Can you work these out from the model? Positions are in its coordinate system, mm. Face numbers are marked on the shaded views. A direction names the side the tool comes from. Give positions to 0.01 mm unless a question says otherwise; leave off trailing zeros. Write each loop counter-clockwise with the first axis right and the second up, starting at its lowest first coordinate (ties: lowest second). Pieces come first, ordered by that corner, then holes. Notation, with made-up numbers: (13, 44.25) - (47, 44.25) arc R13 cw to (47, 63.25) - close; hole circle Ø1 at (48.25, -18.5). An arc over 180 degrees is marked (long way). Return JSON: item names as keys, results as strings. Group by question number.
from build123d import *

# Parameters (mm, degrees)
RESSALTO_EXTRUS_O2_DEPTH      = 30
RESSALTO_EXTRUS_O3_START      = 3
RESSALTO_EXTRUS_O3_DEPTH      = 3
RESSALTO_EXTRUS_O4_DEPTH      = 3
RESSALTO_EXTRUS_O4_DEPTH_BACK = 10
CORTE_EXTRUS_O1_DEPTH         = 10
CORTE_EXTRUS_O2_REACH         = 83.702
FILETE1_START                 = -19.773073923
FILETE1_DEPTH                 = 36.75
FILETE1_START_2               = -13.40159992
FILETE1_2_DEPTH               = 59
ESBO_O10_R                    = 1.5
CORTE_EXTRUS_O3_DEPTH         = 10
CORTE_EXTRUS_O4_DEPTH         = 10
FILETE2_R                     = 2


with BuildPart() as part:
    # Esboço2 → Ressalto-extrusão2 (new body)
    with BuildSketch(Plane(origin=(0, 0, 0), x_dir=(0, 0, -1), z_dir=(1, 0, 0))):
        with BuildLine():
            Line((2.90159992, -0.062465938), (-35.09840008, -0.062465938))
            Line((-35.09840008, -0.062465938), (-39.886084903, -0.062465938))
            ThreePointArc((-39.886084903, -0.062465938), (-45.202180234, 1.467638524), (-48.891439328, 5.589707975))
            ThreePointArc((-48.891439328, 5.589707975), (-52.096536948, 9.772081499), (-56.69840008, 12.338743681))
            ThreePointArc((-56.69840008, 12.338743681), (-59.373224015, 11.895603401), (-60.59840008, 9.476926077))
            Line((-60.59840008, 9.476926077), (-60.59840008, 20.976926077))
            ThreePointArc((-60.59840008, 20.976926077), (-59.719720424, 23.09824642), (-57.59840008, 23.976926077))
            Line((-57.59840008, 23.976926077), (25.40159992, 23.976926077))
            ThreePointArc((25.40159992, 23.976926077), (27.522920263, 23.09824642), (28.40159992, 20.976926077))
            Line((28.40159992, 20.976926077), (28.40159992, 9.476926077))
            ThreePointArc((28.40159992, 9.476926077), (27.176423855, 11.895603401), (24.50159992, 12.338743681))
            ThreePointArc((24.50159992, 12.338743681), (19.899736788, 9.772081499), (16.694639168, 5.589707975))
            ThreePointArc((16.694639168, 5.589707975), (13.005380073, 1.467638524), (7.689284743, -0.062465938))
            Line((7.689284743, -0.062465938), (2.90159992, -0.062465938))
        make_face()
    extrude(amount=RESSALTO_EXTRUS_O2_DEPTH)

    # Esboço3 → Ressalto-extrusão3 (add)
    with BuildSketch(Plane.ZY.offset(RESSALTO_EXTRUS_O3_START)):
        with BuildLine():
            Line((60.59840008, 15.226926077), (60.59840008, 20.976926077))
            ThreePointArc((60.59840008, 20.976926077), (59.719720424, 23.09824642), (57.59840008, 23.976926077))
            Line((57.59840008, 23.976926077), (16.09840008, 23.976926077))
            Line((16.09840008, 23.976926077), (-25.40159992, 23.976926077))
            ThreePointArc((-25.40159992, 23.976926077), (-27.522920263, 23.09824642), (-28.40159992, 20.976926077))
            Line((-28.40159992, 20.976926077), (-28.40159992, 15.226926077))
            Line((-28.40159992, 15.226926077), (-28.40159992, -16.773073923))
            ThreePointArc((-28.40159992, -16.773073923), (-27.522920263, -18.894394267), (-25.40159992, -19.773073923))
            Line((-25.40159992, -19.773073923), (57.59840008, -19.773073923))
            ThreePointArc((57.59840008, -19.773073923), (59.719720424, -18.894394267), (60.59840008, -16.773073923))
            Line((60.59840008, -16.773073923), (60.59840008, 15.226926077))
        make_face()
    extrude(amount=-RESSALTO_EXTRUS_O3_DEPTH)

    # Esboço4 → Ressalto-extrusão4 (add, two sides: drawn at the far end of the back side and taken through both)
    with BuildSketch(Plane(origin=(30, 0, 0), x_dir=(0, 0, -1), z_dir=(1, 0, 0)).offset(-RESSALTO_EXTRUS_O4_DEPTH_BACK)):
        with BuildLine():
            Line((-16.09840008, 23.976926077), (25.40159992, 23.976926077))
            ThreePointArc((25.40159992, 23.976926077), (27.522920263, 23.09824642), (28.40159992, 20.976926077))
            Line((28.40159992, 20.976926077), (28.40159992, 15.226926077))
            Line((28.40159992, 15.226926077), (28.40159992, -16.773073923))
            ThreePointArc((28.40159992, -16.773073923), (27.522920263, -18.894394267), (25.40159992, -19.773073923))
            Line((25.40159992, -19.773073923), (-57.59840008, -19.773073923))
            ThreePointArc((-57.59840008, -19.773073923), (-59.719720424, -18.894394267), (-60.59840008, -16.773073923))
            Line((-60.59840008, -16.773073923), (-60.59840008, 15.226926077))
            Line((-60.59840008, 15.226926077), (-60.59840008, 20.976926077))
            ThreePointArc((-60.59840008, 20.976926077), (-59.719720424, 23.09824642), (-57.59840008, 23.976926077))
            Line((-57.59840008, 23.976926077), (-16.09840008, 23.976926077))
        make_face()
    extrude(amount=RESSALTO_EXTRUS_O4_DEPTH + RESSALTO_EXTRUS_O4_DEPTH_BACK)

    # Esboço8 → Corte-extrusão1 (cut)
    with BuildSketch(Plane(origin=(33, 0, 0), x_dir=(0, 0, -1), z_dir=(1, 0, 0))):
        with BuildLine():
            Line((-43.59840008, -2.773073923), (11.40159992, -2.773073923))
            ThreePointArc((11.40159992, -2.773073923), (12.815813482, -3.358860361), (13.40159992, -4.773073923))
            Line((13.40159992, -4.773073923), (13.40159992, -10.773073923))
            ThreePointArc((13.40159992, -10.773073923), (12.815813482, -12.187287486), (11.40159992, -12.773073923))
            Line((11.40159992, -12.773073923), (-43.59840008, -12.773073923))
            ThreePointArc((-43.59840008, -12.773073923), (-45.012613643, -12.187287486), (-45.59840008, -10.773073923))
            Line((-45.59840008, -10.773073923), (-45.59840008, -4.773073923))
            ThreePointArc((-45.59840008, -4.773073923), (-45.012613643, -3.358860361), (-43.59840008, -2.773073923))
        make_face()
        with BuildLine():
            Line((-43.59840008, 6.976926077), (11.40159992, 6.976926077))
            ThreePointArc((11.40159992, 6.976926077), (12.815813482, 7.562712514), (13.40159992, 8.976926077))
            Line((13.40159992, 8.976926077), (13.40159992, 14.976926077))
            ThreePointArc((13.40159992, 14.976926077), (12.815813482, 16.391139639), (11.40159992, 16.976926077))
            Line((11.40159992, 16.976926077), (-43.59840008, 16.976926077))
            ThreePointArc((-43.59840008, 16.976926077), (-45.012613643, 16.391139639), (-45.59840008, 14.976926077))
            Line((-45.59840008, 14.976926077), (-45.59840008, 8.976926077))
            ThreePointArc((-45.59840008, 8.976926077), (-45.012613643, 7.562712514), (-43.59840008, 6.976926077))
        make_face()
    extrude(amount=-CORTE_EXTRUS_O1_DEPTH, mode=Mode.SUBTRACT)

    # Corte-extrusão2: up to this face of the body (flat: up to its plane)
    corte_extrus_o2_end = Plane(part.part.faces().sort_by_distance((28, 16.976926077, 16.09840008))[0])
    # Esboço9 → Corte-extrusão2 (cut, up to the picked face)
    with BuildSketch(Plane(origin=(0, -19.773073923, 0), x_dir=(-1, 0, 0), z_dir=(0, -1, 0)), mode=Mode.PRIVATE) as corte_extrus_o2_sk1:
        with BuildLine():
            Line((-25, 13.40159992), (-28, 13.40159992))
            ThreePointArc((-28, 13.40159992), (-29.414213562, 12.815813482), (-30, 11.40159992))
            Line((-30, 11.40159992), (-30, -43.59840008))
            ThreePointArc((-30, -43.59840008), (-29.414213562, -45.012613643), (-28, -45.59840008))
            Line((-28, -45.59840008), (-25, -45.59840008))
            ThreePointArc((-25, -45.59840008), (-23.585786438, -45.012613643), (-23, -43.59840008))
            Line((-23, -43.59840008), (-23, 11.40159992))
            ThreePointArc((-23, 11.40159992), (-23.585786438, 12.815813482), (-25, 13.40159992))
        make_face()
    corte_extrus_o2_tool1 = split(extrude(corte_extrus_o2_sk1.sketch, amount=-CORTE_EXTRUS_O2_REACH, mode=Mode.PRIVATE), bisect_by=corte_extrus_o2_end, keep=Keep.BOTH, mode=Mode.PRIVATE)
    add(corte_extrus_o2_tool1.solids().sort_by(Axis((26.5, -19.773074, 16.0984), (0, 1, 0)))[0], mode=Mode.SUBTRACT)

    # Filete1: read off the stored shape, not the designer's step
    # Filete1 outline → Filete1 (add)
    with BuildSketch(Plane(origin=(0, 0, 0), x_dir=(1, 0, 0), z_dir=(0, 1, 0)).offset(FILETE1_START)):
        with BuildLine():
            ThreePointArc((25, -45.59840008), (23.585786437, -45.012613642), (23, -43.59840008))
            Line((23, -43.59840008), (23, -45.59840008))
            Line((23, -45.59840008), (25, -45.59840008))
        make_face()
        with BuildLine():
            ThreePointArc((23, 11.40159992), (23.585786438, 12.815813482), (25, 13.40159992))
            Line((25, 13.40159992), (23, 13.40159992))
            Line((23, 13.40159992), (23, 11.40159992))
        make_face()
    extrude(amount=FILETE1_DEPTH)

    # Filete1 2 outline → Filete1 2 (add)
    with BuildSketch(Plane.XY.offset(FILETE1_START_2)):
        with BuildLine():
            ThreePointArc((23, 14.976926077), (23.585786438, 16.391139639), (25, 16.976926077))
            Line((25, 16.976926077), (23, 16.976926077))
            Line((23, 16.976926077), (23, 14.976926077))
        make_face()
    extrude(amount=FILETE1_2_DEPTH)

    # Esboço10 → Corte-extrusão3 (cut)
    with BuildSketch(Plane(origin=(0, 0, 0), x_dir=(0, 0, -1), z_dir=(1, 0, 0))):
        with Locations((-55.59840008, 6.338743681)):
            Circle(ESBO_O10_R)
        with Locations((23.40159992, 6.338743681)):
            Circle(ESBO_O10_R)
        with Locations((-16.09840008, -8.562465938)):
            Circle(ESBO_O10_R)
    extrude(amount=-CORTE_EXTRUS_O3_DEPTH, mode=Mode.SUBTRACT)

    # Esboço12 → Corte-extrusão4 (cut)
    with BuildSketch(Plane(origin=(0, 0, 0), x_dir=(0, 0, -1), z_dir=(1, 0, 0))):
        with BuildLine():
            Line((-31.59840008, -2.862465938), (-25.59840008, -2.862465938))
            ThreePointArc((-25.59840008, -2.862465938), (-24.184186518, -3.448252375), (-23.59840008, -4.862465938))
            Line((-23.59840008, -4.862465938), (-23.59840008, -14.773073923))
            ThreePointArc((-23.59840008, -14.773073923), (-24.184186518, -16.187287486), (-25.59840008, -16.773073923))
            Line((-25.59840008, -16.773073923), (-31.59840008, -16.773073923))
            ThreePointArc((-31.59840008, -16.773073923), (-33.012613643, -16.187287486), (-33.59840008, -14.773073923))
            Line((-33.59840008, -14.773073923), (-33.59840008, -4.862465938))
            ThreePointArc((-33.59840008, -4.862465938), (-33.012613643, -3.448252375), (-31.59840008, -2.862465938))
        make_face()
        with BuildLine():
            Line((-6.59840008, -2.862465938), (-0.59840008, -2.862465938))
            ThreePointArc((-0.59840008, -2.862465938), (0.815813482, -3.448252375), (1.40159992, -4.862465938))
            Line((1.40159992, -4.862465938), (1.40159992, -14.773073923))
            ThreePointArc((1.40159992, -14.773073923), (0.815813482, -16.187287486), (-0.59840008, -16.773073923))
            Line((-0.59840008, -16.773073923), (-6.59840008, -16.773073923))
            ThreePointArc((-6.59840008, -16.773073923), (-8.012613643, -16.187287486), (-8.59840008, -14.773073923))
            Line((-8.59840008, -14.773073923), (-8.59840008, -4.862465938))
            ThreePointArc((-8.59840008, -4.862465938), (-8.012613643, -3.448252375), (-6.59840008, -2.862465938))
        make_face()
    extrude(amount=-CORTE_EXTRUS_O4_DEPTH, mode=Mode.SUBTRACT)

    # Filete2
    filete2_edges = [part.edges().sort_by_distance(p)[0] for p in [
        (-3, 2.101926077, 60.59840008),
        (-3, 23.09824642, 59.719720424),
        (-3, 23.976926077, 16.09840008),
        (-3, 23.09824642, -27.522920263),
        (-3, 2.101926077, -28.40159992),
        (-3, -18.894394267, -27.522920263),
        (-3, -19.773073923, 16.09840008),
        (-3, -18.894394267, 59.719720424),
    ]]
    fillet(filete2_edges, radius=FILETE2_R)


solid = part.part
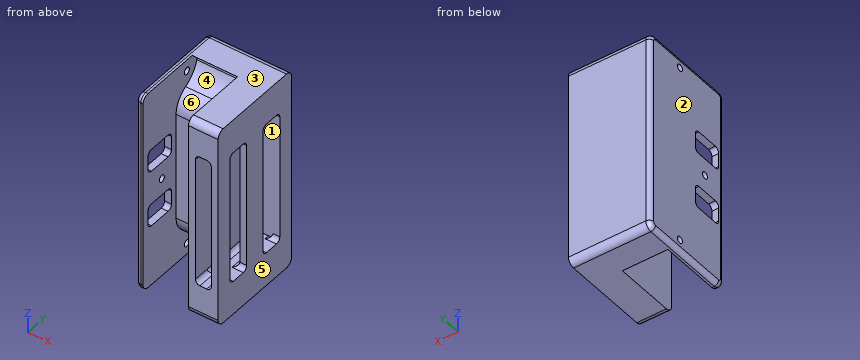
1) Imagine slicing it at D-D, the plane x = 14. Write out the boundary of the cut face in (y, z), and give its area (3 significant figures).
2) Imagine slicing it at C-C, the plane z = 36.5. Write out the boundary of the cut face in (x, y), and give its area (3 significant figures).
3) Imagine slicing it at A-A, the plane z = 5. Write out the boundary of the cut face in (x, y).
4) Will these pins go through, and if not, where does the flat tip stop? pin 1 Ø1.5 at (x, y) = (-2, -9.5) entering from +Z; pin 2 Ø16 at (x, z) = (10.5, 11) entering from -Y; pin 3 Ø0.9 at (x, z) = (-2, 28.5) entering from -Y.
5) I need wall thicknesses on line 1 along X through (y, z) = (-2.5, -9.5); line 2 along X through (y, z) = (-2, 46); line 3 along X through (y, z) = (1, 23.5). Which ranges of each line are inside material? Lowest first, please.
6) On a 3-axis mill with a long thin cutter (end or side, diameter ignored), from which of +Z, -Z, +X, -X, +Y, -Y can I reach the whole of each face in a straight line? I mean the marked faces 4, 5 and 6. Say none if no direction works.
7) Imagine slicing it at B-B, the plane y = -6. Write out the boundary of the cut face in (x, z).
8) We'd pull the mould along Z, two halves only. Please class the marked faces 1, 2 and 3: pulls with the +Z half, pulls with the -Z half, needs draft (parallel to the pull), parting line crosses it, or undercut.
Resolved:
{
 "1": {"outline": "(-0.06, -7.69) arc R10 ccw to (5.59, -16.69) arc R13 cw to (12.34, -24.5) arc R3 cw to (9.48, -28.4) - (20.98, -28.4) arc R3 ccw to (23.98, -25.4) - (23.98, 57.6) arc R3 ccw to (20.98, 60.6) - (9.48, 60.6) arc R3 cw to (12.34, 56.7) arc R13 cw to (5.59, 48.89) arc R10 ccw to (-0.06, 39.89) - close", "area": "1,860 mm^2"},
 "2": {"outline": "(-3, -17.77) arc R2 ccw to (-1, -19.77) - (0, -19.77) - (0, -0.06) - (20, -0.06) - (20, -19.77) - (23, -19.77) - (23, 14.98) arc R2 cw to (25, 16.98) - (33, 16.98) - (33, 23.98) - (-1, 23.98) arc R2 ccw to (-3, 21.98) - close; (30, -19.77) - (33, -19.77) - (33, -12.77) - (30, -12.77) - close; (30, -2.77) - (33, -2.77) - (33, 6.98) - (30, 6.98) - close", "area": "863 mm^2"},
 "3": {"outline": "(-3, -17.77) arc R2 ccw to (-1, -19.77) - (0, -19.77) - (0, -16.77) - (-3, -16.77) - close; (-3, -2.86) - (0, -2.86) - (0, -0.06) - (20, -0.06) - (20, -19.77) - (23, -19.77) - (23, 14.98) arc R2 cw to (25, 16.98) - (33, 16.98) - (33, 23.98) - (-1, 23.98) arc R2 ccw to (-3, 21.98) - close; (30, -19.77) - (33, -19.77) - (33, -12.77) - (30, -12.77) - close; (30, -2.77) - (33, -2.77) - (33, 6.98) - (30, 6.98) - close"},
 "4": {"pin 1": "z = 60.58", "pin 2": "y = -0.06", "pin 3": "y = -19.7"},
 "5": {"line 1": "-3 to 0, 20 to 23, 30 to 33", "line 2": "-3 to 0, 20 to 33", "line 3": "-3 to 23, 30 to 33"},
 "6": {"face 4": "-Y", "face 5": "+Z, -Z, +X, +Y, -Y", "face 6": "+Z, -Y"},
 "7": {"outline": "(-3, -26.4) arc R2 ccw to (-1, -28.4) - (0, -28.4) - (0, -1.4) - (-3, -1.4) - close; (-3, 8.6) - (0, 8.6) - (0, 23.6) - (-3, 23.6) - close; (-3, 33.6) - (0, 33.6) - (0, 60.6) - (-1, 60.6) arc R2 ccw to (-3, 58.6) - close; (20, -28.4) - (33, -28.4) - (33, -13.4) - (25, -13.4) arc R2 cw to (23, -11.4) - (23, 43.6) arc R2 cw to (25, 45.6) - (33, 45.6) - (33, 60.6) - (20, 60.6) - close"},
 "8": {"face 1": "undercut", "face 2": "needs draft", "face 3": "pulls with the +Z half"}
}
